Autodesk Inventor part; units mm, degrees
sketch "Sketch1" plane through (0, 0, 0) normal (0, 0, 1) x (1, 0, 0)
  line L0 (0, 2.8582) -> (0, -2.8582) construction
  line L1 (-5.7775, 0) -> (5.7775, 0) construction
  line L2 (-35.25, -6.5) -> (35.25, -6.5)
  line L3 (35.25, -6.5) -> (35.25, 6.5)
  line L4 (35.25, 6.5) -> (-35.25, 6.5)
  line L5 (-35.25, 6.5) -> (-35.25, -6.5)
  line L6 (-35.25, -6.5) -> (35.25, 6.5) construction
  line L7 (35.25, -6.5) -> (-35.25, 6.5) construction
  line L8 (-37.75, 9) -> (37.75, 9)
  line L9 (37.75, 9) -> (37.75, -9)
  line L10 (37.75, -9) -> (-37.75, -9)
  line L11 (-37.75, -9) -> (-37.75, 9)
  line L12 (-37.75, 9) -> (37.75, -9) construction
  line L13 (37.75, 9) -> (-37.75, -9) construction
  point P0 (0, 0)
  point P1 (0, 0)
  dimension "d0" = 70.5
  dimension "d1" = 13
  dimension "d2" = 2.5
  dimension "d3" = 2.5
extrude "Extrusion1" add sketch "Sketch1" along normal blind 130
sketch "Sketch2" plane through (0, 0, 0) normal (0, 0, -1) x (-1, 0, 0)
  line L0 (-35.25, -6.5) -> (35.25, -6.5)
  line L1 (35.25, -6.5) -> (35.25, 6.5)
  line L2 (35.25, 6.5) -> (-35.25, 6.5)
  line L3 (-35.25, 6.5) -> (-35.25, -6.5)
  line L4 (37.75, 9) -> (37.75, -9)
  line L5 (37.75, -9) -> (-37.75, -9)
  line L6 (-37.75, -9) -> (-37.75, 9)
  line L7 (-37.75, 9) -> (37.75, 9)
  point P0 (0, 0)
extrude "Extrusion2" add sketch "Sketch2" along normal blind 2.5 contours L3 L2 L1 L0 | L4 L5 L6 L7
sketch "Sketch3" plane through (-37.75, -9, 130) normal (0, -1, 0) x (1, 0, 0)
  line L0 (75.5, -132.5) -> (0, -132.5)
  line L1 (0, -132.5) -> (0, 0)
  line L2 (0, 0) -> (75.5, 0)
  line L3 (75.5, 0) -> (75.5, -132.5)
  line L4 (0, -32.5) -> (75.5, -32.5)
  line L5 (2.5, -130) -> (2.5, 0)
  line L6 (73, -130) -> (73, 0)
  point P0 (37.75, -130)
  point P1 (73, -32.5)
  point P2 (2.5, -32.5)
  dimension "d8" = 100
extrude "Extrusion3" cut sketch "Sketch3" against normal up to surface (2.5 mm away) contours L4 L5 L2 L6
fillet "Fillet1" radius 2 1 edges at (0, -9, 97.5)
fillet "Fillet2" radius 2 2 edges at (-37.75, -9, 63.75) (37.75, -9, 63.75)
equation "\"d3\" = d2"
properties part number "Powerbank Holder" material "S235"
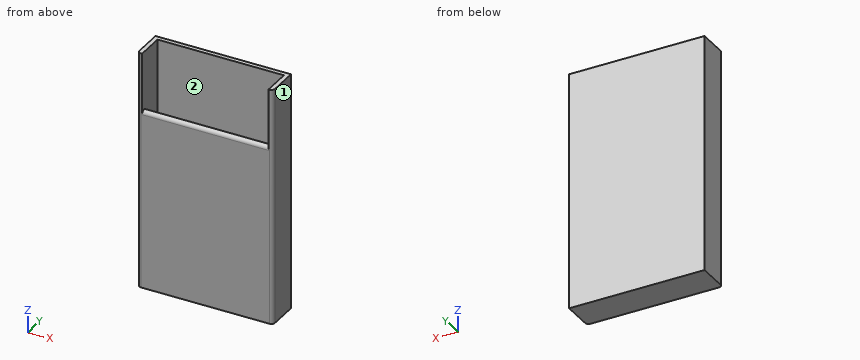
The model under review builds one solid part; all positions refer to its coordinate system, in mm. Face numbers are marked on the shaded views. A direction names the side the tool comes from. Coordinates: 2 decimals unless noted, no trailing zeros. Order: outer loops, then holes, each group sorted by start corner. A loop starts at its lowest first (then second) coordinate and runs counter-clockwise, first axis right, second up. Notation, with made-up numbers: (78.25, 7.25) -> (114.25, 7.25) arc R10 cw to (114.25, 14.25) -> close; hole circle Ø6 at (60, 36). An arc over 180 degrees is marked (long way). Answer in a Markdown table with one row per item. Add a question column.
Item 1: We need section A-A on z = 26. Write out the cut boundary in (x, y).
Item 2: To check wall thickness, follow probe 1 along X at (y, z) = (-0.25, 112); probe 2 along Y at (x, z) = (-5, 56); probe 3 along Y at (x, z) = (0, 100). State the ranges of each line that lie inside material, in increasing order.
Item 3: Clearance check with a flat-ended pin moving along its axis: pin 1 (4 mm diameter, centred on x = 11.5, y = -0.5, fed in from +Z). State where the tip first meets the part, or that it passes through.
Item 4: Machinability: for the marked faces 1 and 2, which of the approach directions +Z, -Z, +X, -X, +Y, -Y give a long, thin tool a straight path to every point of the face, cutting with its end or side? Answer none if there is none.
Item 5: We need section D-D on z = 107. Write out the cut boundary in (x, y), plus the area to 3 significant figures.
Item 6: We need section C-C on y = 4.5. Write out the cut boundary in (x, z), plus the area to 3 significant figures.
Item 7: We need section B-B on x = 19. Write out the cut boundary in (y, z), plus the area to 3 significant figures.
Final values:
| question | item | result |
|---|---|---|
| 1 | outline | (-37.75, -7) arc R2 ccw to (-35.75, -9) -> (35.75, -9) arc R2 ccw to (37.75, -7) -> (37.75, 9) -> (-37.75, 9) -> close; hole (-35.25, -6.5) -> (35.25, -6.5) -> (35.25, 6.5) -> (-35.25, 6.5) -> close |
| 2 | probe 1 | x = -37.75 to -35.25, 35.25 to 37.75 |
| 2 | probe 2 | y = -9 to -6.5, 6.5 to 9 |
| 2 | probe 3 | y = 6.5 to 9 |
| 3 | pin 1 | stops at z = 0 |
| 4 | face 1 | +Z, -Z, +X, +Y, -Y |
| 4 | face 2 | +Z |
| 5 | outline | (-37.75, -7) arc R2 ccw to (-35.75, -9) -> (-35.25, -9) -> (-35.25, 6.5) -> (35.25, 6.5) -> (35.25, -9) -> (35.75, -9) arc R2 ccw to (37.75, -7) -> (37.75, 9) -> (-37.75, 9) -> close |
| 5 | area | 265 mm2 |
| 6 | outline | (-37.75, -2.5) -> (37.75, -2.5) -> (37.75, 130) -> (35.25, 130) -> (35.25, 0) -> (-35.25, 0) -> (-35.25, 130) -> (-37.75, 130) -> close |
| 6 | area | 839 mm2 |
| 7 | outline | (-9, -2.5) -> (9, -2.5) -> (9, 130) -> (6.5, 130) -> (6.5, 0) -> (-6.5, 0) -> (-6.5, 97.5) -> (-7, 97.5) arc R2 ccw to (-9, 95.5) -> close |
| 7 | area | 613 mm2 |
